Source: CAD feature listing. Evaluate the final solid. Frame: model axes, mm. A direction names the side the tool comes from. Give positions to 0.01 mm unless a question says otherwise; leave off trailing zeros. Order: outer loops, then holes, each group sorted by start corner. A loop starts at its lowest first (then second) coordinate and runs counter-clockwise, first axis right, second up. Notation, with made-up numbers: (-4.75, -23) - (18.25, -23) arc R15 ccw to (18.25, 6) - close; hole circle Ø2 at (62.25, 65.25). An arc over 180 degrees is marked (long way). Answer as CSV lines item,"result".
```python
from build123d import *

# Parameters (mm, degrees)
EXTRUDE_2_DEPTH = 8
CHAMFER_1_SIZE  = 1
SKETCH_5_R      = 2.5
EXTRUDE_3_DEPTH = 2
FILLET_3_R      = 1


with BuildPart() as part:
    # 草图2 → 旋转1 (revolve)
    with BuildSketch(Plane(origin=(0, 0, 0), x_dir=(0, 0, -1), z_dir=(1, 0, 0)), mode=Mode.PRIVATE) as revolve_1_sk:
        Polygon((3.53910226, 2.5), (3.53910226, 8), (3.03910226, 8.5), (-5.96089774, 8.5), (-6.46089774, 8), (-6.46089774, 7.5), (-31.46089774, 4.5), (-31.46089774, 2.5), align=None)
    revolve(revolve_1_sk.sketch.rotate(Axis((0, 0, 0), (0, 0, -1)), 90), axis=Axis((0, 0, 0), (0, 0, -1)))

    # 草图4 → 凸台-拉伸2 (add)
    with BuildSketch(Plane(origin=(0, 0, -3.53910226), x_dir=(-1, 0, 0), z_dir=(0, 0, -1))):
        Polygon((0, 8), (-6.92820323, 4), (-6.92820323, -4), (0, -8), (6.92820323, -4), (6.92820323, 4), align=None)
    extrude(amount=EXTRUDE_2_DEPTH)

    # 倒角1
    chamfer_1_edges = [part.edges().sort_by_distance(p)[0] for p in [
        (-3.464101615, 6, -11.53910226),
        (3.464101615, 6, -11.53910226),
        (6.92820323, 0, -11.53910226),
        (3.464101615, -6, -11.53910226),
        (-3.464101615, -6, -11.53910226),
        (-6.92820323, 0, -11.53910226),
    ]]
    chamfer(chamfer_1_edges, length=CHAMFER_1_SIZE)

    # 草图5 → 凸台-拉伸3 (add, symmetric)
    with BuildSketch(Plane(origin=(0, 0, 0), x_dir=(1, 0, 0), z_dir=(0, 1, 0))):
        with BuildLine():
            Line((-4.25, 11.53910226), (4.25, 11.53910226))
            Line((4.25, 11.53910226), (4.25, 17.53910226))
            ThreePointArc((4.25, 17.53910226), (3.078427125, 20.367529385), (0.25, 21.53910226))
            Line((0.25, 21.53910226), (-0.25, 21.53910226))
            ThreePointArc((-0.25, 21.53910226), (-3.078427125, 20.367529385), (-4.25, 17.53910226))
            Line((-4.25, 17.53910226), (-4.25, 11.53910226))
        make_face()
        with Locations(Location((0, 17.53910226, 0), (0, 0, 270))):
            Circle(SKETCH_5_R, mode=Mode.SUBTRACT)
    extrude(amount=EXTRUDE_3_DEPTH, both=True)

    # 圆角3
    fillet_3_edges = [part.edges().sort_by_distance(p)[0] for p in [
        (-4.25, -2, -14.53910226),
        (4.25, -2, -14.53910226),
        (3.078427125, -2, -20.367529385),
        (0, -2, -21.53910226),
        (-3.078427125, -2, -20.367529385),
    ]]
    fillet(fillet_3_edges, radius=FILLET_3_R)
    fillet_3_2_edges = [part.edges().sort_by_distance(p)[0] for p in [
        (-4.25, 2, -14.53910226),
        (4.25, 2, -14.53910226),
        (3.078427125, 2, -20.367529385),
        (0, 2, -21.53910226),
        (-3.078427125, 2, -20.367529385),
    ]]
    fillet(fillet_3_2_edges, radius=FILLET_3_R)
    fillet_3_3_edges = [part.edges().sort_by_distance(p)[0] for p in [
        (0, 2, -11.53910226),
    ]]
    fillet(fillet_3_3_edges, radius=FILLET_3_R)
    # the kernel refuses this fillet: 1 mm, written as the material it takes off along each edge
    with BuildSketch(Plane(origin=(0, 2, -17.53910226), x_dir=(0, 0, 1), z_dir=(-1, 0, 0))) as fillet_3_4_piece_1:
        with BuildLine():
            CenterArc((2.5 + FILLET_3_R, -FILLET_3_R), FILLET_3_R, 90, 90)
            Line((2.5, -FILLET_3_R), (2.5 - FILLET_3_R * 0.02, -FILLET_3_R))
            Line((2.5 - FILLET_3_R * 0.02, -FILLET_3_R), (2.5 - FILLET_3_R * 0.02, FILLET_3_R * 0.02))
            Line((2.5 - FILLET_3_R * 0.02, FILLET_3_R * 0.02), (2.5 + FILLET_3_R, FILLET_3_R * 0.02))
            Line((2.5 + FILLET_3_R, FILLET_3_R * 0.02), (2.5 + FILLET_3_R, 0))
        make_face()
    revolve(axis=Axis((0, 2, -17.53910226), (0, 1, 0)), mode=Mode.SUBTRACT)
    # the kernel refuses this fillet: 1 mm, written as the material it takes off along each edge
    with BuildSketch(Plane(origin=(0, -2, -17.53910226), x_dir=(0, 0, 1), z_dir=(-1, 0, 0))) as fillet_3_5_piece_1:
        with BuildLine():
            CenterArc((2.5 + FILLET_3_R, FILLET_3_R), FILLET_3_R, 180, 90)
            Line((2.5, FILLET_3_R), (2.5 - FILLET_3_R * 0.02, FILLET_3_R))
            Line((2.5 - FILLET_3_R * 0.02, FILLET_3_R), (2.5 - FILLET_3_R * 0.02, -FILLET_3_R * 0.02))
            Line((2.5 - FILLET_3_R * 0.02, -FILLET_3_R * 0.02), (2.5 + FILLET_3_R, -FILLET_3_R * 0.02))
            Line((2.5 + FILLET_3_R, -FILLET_3_R * 0.02), (2.5 + FILLET_3_R, 0))
        make_face()
    revolve(axis=Axis((0, -2, -17.53910226), (0, 1, 0)), mode=Mode.SUBTRACT)


solid = part.part
```
(1) Mould query, pull axis Y, two halves, no side actions, for faces 6 (the cylindrical face through (-2.5, -0.1, 13.7)), 7 (the flat face through (4, 6, -3.539)), 8 (the flat face through (-3.416, -6.028, -6.99)), 9 (the cylindrical face through (3.965, 1.699, -15.074)). Classes: released by +Y, released by -Y, zero draft, split by the parting line, or undercut.
Completed:
face 6,"undercut"
face 7,"zero draft"
face 8,"released by -Y"
face 9,"released by +Y"
(2) Access query for faces 1 (the flat face through (0, 2, -13.6)), 2 (the flat face through (3.513, -5.972, -6.99)), 3 (the flat face through (6.928, 0, -7)), 4 (the flat face through (-7.3, -0.1, -3.539)), 5 (the cylindrical face through (-3.965, 1.699, -15.004)). Directions: +Z, -Z, +X, -X, +Y, -Y. A direction counts if a zero-diameter tool reaches every point of the face in a straight line with its end or side. Return the directions, or none.
Completed:
face 1,"-Z, +X, -X, +Y"
face 2,"-Z, +X, -Y"
face 3,"-Z, +X, +Y, -Y"
face 4,"-Z, -X, +Y, -Y"
face 5,"-Z, -X, +Y"
(3) Ray query, line 1 (Y direction, x = 0, z = 5); line 2 (X direction, y = 1, z = -7); line 3 (Y direction, x = 0, z = 9.5). Return the intervals inside material, ascending. Write a range as from..to.
Completed:
line 1,"-8.5..-2.5, 2.5..8.5"
line 2,"-6.93..6.93"
line 3,"-7.14..-2.5, 2.5..7.14"
(4) Contact query for flat-ended pins moving along their axis: pin 1 (1.5 mm diameter, centred on x = -0.5, y = 1, fed in from +Z); pin 2 (2 mm diameter, centred on x = -4.5, y = -7, fed in from -Z); pin 3 (3.5 mm diameter, centred on x = -2, y = -3, fed in from -Z). Output: stop coordinate, or through.
Completed:
pin 1,"z = -3.54"
pin 2,"z = -3.54"
pin 3,"z = -21.32"
(5) Cut plane B-B (z = 4.5). Return loops of the section in (x, y), then the cut area to 3 significant figures.
Completed:
outline,"circle Ø17 at (0, 0); hole circle Ø5 at (0, 0)"
area,"207 mm²"
